For this review, take the finished solid that the model builds, in its own axes (mm). Coordinates: 2 decimals unless noted, no trailing zeros. Write each loop counter-clockwise with the first axis right and the second up, starting at its lowest first coordinate (ties: lowest second). Pieces come first, ordered by that corner, then holes.
1) We need section D-D on y = 229. Write out the cut boundary in (x, z).
2) We need section C-C on z = 41.5. Write out the cut boundary in (x, y).
3) To check wall thickness, follow line 1 along Y through (x, z) = (2181, 280); line 2 along Z through (x, y) = (1688.5, 131); line 3 along Y through (x, z) = (1831, 144). State the ranges of each line that lie inside material, in increasing order.
4) Insertion check: P1, Ø6, axis at x = 616.5, y = 173.5, coming from the -Z side; P2, Ø8, axis at x = 1564.5, y = 34.5, coming from the -Z side; P3, Ø5, axis at x = 449.5, y = 135.5, coming from the -Z side; P4, Ø8, axis at y = 146, z = 490.5, coming from the -X side. Each pin has a flat end and moves straight along its axis. Give the tip position at first contact, or say it passes through.
5) We need section A-A on x = 716. Write out the cut boundary in (y, z).
6) Mouldability with a two-part tool opening along X and no side actions: class faces 1 (the face through (1233, 284, 386)), 2 (the face through (2500, 140, 247)), 3 (the face through (1233, 144, 480)) as pulls with the +X half, pulls with the -X half, needs draft (parallel to the pull), parting line crosses it, or undercut.
7) We need section B-B on y = 139. Write out the cut boundary in (x, z).
from build123d import *

# Parameters (mm, degrees)
SKETCH1_W           = 2500
SKETCH1_H           = 284
BOSS_EXTRUDE1_DEPTH = 500
FILLET1_R           = 10
SKETCH2_W           = 2436
SKETCH2_H           = 220
CUT_EXTRUDE1_DEPTH  = 20
FILLET2_R           = 2
CUT_EXTRUDE2_REACH  = 2567.279


with BuildPart() as part:
    # Sketch1 → Boss-Extrude1 (new body)
    with BuildSketch(Plane.XY):
        with Locations((1250, 142)):
            Rectangle(SKETCH1_W, SKETCH1_H)
    extrude(amount=BOSS_EXTRUDE1_DEPTH)

    # Fillet1
    fillet1_edges = [part.edges().sort_by_distance(p)[0] for p in [
        (2500, 142, 500),
        (1250, 284, 500),
        (0, 142, 500),
        (1250, 284, 0),
        (2500, 142, 0),
        (1250, 0, 0),
        (0, 142, 0),
        (0, 284, 250),
        (2500, 284, 250),
        (2500, 0, 250),
        (0, 0, 250),
        (1250, 0, 500),
    ]]
    fillet(fillet1_edges, radius=FILLET1_R)

    # Sketch2 → Cut-Extrude1 (cut)
    with BuildSketch(Plane.XY.offset(500)):
        with Locations((1250, 142)):
            Rectangle(SKETCH2_W, SKETCH2_H)
    extrude(amount=-CUT_EXTRUDE1_DEPTH, mode=Mode.SUBTRACT)

    # Fillet2
    fillet2_edges = [part.edges().sort_by_distance(p)[0] for p in [
        (2468, 142, 480),
        (2468, 252, 490),
        (1250, 32, 480),
        (2468, 32, 490),
        (32, 142, 480),
        (32, 32, 490),
        (1250, 252, 480),
        (32, 252, 490),
        (2468, 142, 500),
        (1250, 252, 500),
        (32, 142, 500),
        (1250, 32, 500),
    ]]
    fillet(fillet2_edges, radius=FILLET2_R)

    # Cut-Extrude2: up to this face of the body (flat: up to its plane)
    cut_extrude2_end = Plane(part.part.faces().sort_by_distance((2500, 142, 250))[0])
    # Sketch3 → Cut-Extrude2 (cut, up to the picked face)
    with BuildSketch(Plane.ZY, mode=Mode.PRIVATE) as cut_extrude2_sk1:
        with BuildLine():
            Line((284, 284), (0, 284))
            Line((0, 284), (0, 0))
            ThreePointArc((0, 0), (83.181674143, 200.818325857), (284, 284))
        make_face()
    cut_extrude2_tool1 = split(extrude(cut_extrude2_sk1.sketch, amount=-CUT_EXTRUDE2_REACH, mode=Mode.PRIVATE), bisect_by=cut_extrude2_end, keep=Keep.BOTH, mode=Mode.PRIVATE)
    add(cut_extrude2_tool1.solids().sort_by(Axis((0, 220.563505, 63.436495), (1, 0, 0)))[0], mode=Mode.SUBTRACT)


solid = part.part
Result:
1. outline: (0, 116.03) - (2500, 116.03) - (2500, 490) arc R10 ccw to (2490, 500) - (2470, 500) arc R2 ccw to (2468, 498) - (2468, 482) arc R2 cw to (2466, 480) - (34, 480) arc R2 cw to (32, 482) - (32, 498) arc R2 ccw to (30, 500) - (10, 500) arc R10 ccw to (0, 490) - close
2. outline: (0, 10) arc R10 ccw to (10, 0) - (2490, 0) arc R10 ccw to (2500, 10) - (2500, 147.82) - (0, 147.82) - close
3. line 1: y = 0 to 283.97
3. line 2: z = 32.02 to 480
3. line 3: y = 0 to 247.1
4. P1: stops at z = 56.88
4. P2: stops at z = 1.64
4. P3: stops at z = 33.07
4. P4: stops at x = 0
5. outline: (0, 10) arc R10 ccw to (8.42, 0.12) arc R284 ccw to (284, 284) - (284, 490) arc R10 ccw to (274, 500) - (254, 500) arc R2 ccw to (252, 498) - (252, 482) arc R2 cw to (250, 480) - (34, 480) arc R2 cw to (32, 482) - (32, 498) arc R2 ccw to (30, 500) - (10, 500) arc R10 ccw to (0, 490) - close
6. face 1: needs draft
6. face 2: pulls with the +X half
6. face 3: undercut
7. outline: (0, 36.34) - (2500, 36.34) - (2500, 490) arc R10 ccw to (2490, 500) - (2470, 500) arc R2 ccw to (2468, 498) - (2468, 482) arc R2 cw to (2466, 480) - (34, 480) arc R2 cw to (32, 482) - (32, 498) arc R2 ccw to (30, 500) - (10, 500) arc R10 ccw to (0, 490) - close
